Geometry: final body of the model. Coordinates: model frame, mm. A direction names the side the tool comes from. Round coordinates to 2 decimals unless told otherwise and drop trailing zeros. Loops run counter-clockwise (first coordinate to the right, second up) from the corner with the lowest first, then second, coordinate; pieces in that order, holes last. Notation, with made-up numbers: (19.25, 77) - (23.25, 77) arc R37 cw to (23.25, 116) - close; hole circle Ø4 at (54.25, -4). An arc over 180 degrees is marked (long way). Answer as CSV lines item,"result".
from build123d import *

# Parameters (mm, degrees)
SKETCH1_R           = 10.5
SKETCH1_R_2         = 1.5
BOSS_EXTRUDE1_DEPTH = 2.5
SKETCH2_R           = 4.5
SKETCH2_R_2         = 2.5
BOSS_EXTRUDE2_DEPTH = 3
CUT_EXTRUDE1_REACH  = 17.835
SKETCH3_R           = 1


with BuildPart() as part:
    # Sketch1 → Boss-Extrude1 (new body)
    with BuildSketch(Plane(origin=(0, 0, 0), x_dir=(1, 0, 0), z_dir=(0, 1, 0))):
        with Locations(Location((0, 0, 0), (0, 0, 270))):
            Circle(SKETCH1_R)
        with Locations(Location((0, 0, 0), (0, 0, 270))):
            Circle(SKETCH1_R_2, mode=Mode.SUBTRACT)
    extrude(amount=BOSS_EXTRUDE1_DEPTH)

    # Sketch2 → Boss-Extrude2 (add)
    with BuildSketch(Plane(origin=(0, 2.5, 0), x_dir=(1, 0, 0), z_dir=(0, 1, 0))):
        with Locations(Location((0, 0, 0), (0, 0, 270))):
            Circle(SKETCH2_R)
        with Locations(Location((0, 0, 0), (0, 0, 270))):
            Circle(SKETCH2_R_2, mode=Mode.SUBTRACT)
    extrude(amount=BOSS_EXTRUDE2_DEPTH)

    # Sketch3 → Cut-Extrude1 (cut, up to next)
    with BuildSketch(Plane.XZ, mode=Mode.PRIVATE) as cut_extrude1_sk1:
        with Locations(Location((-3.5, 7, 0), (0, 0, 270))):
            Circle(SKETCH3_R)
    cut_extrude1_tool1 = extrude(cut_extrude1_sk1.sketch, amount=-CUT_EXTRUDE1_REACH, mode=Mode.PRIVATE) & part.part
    # Sketch3 → Cut-Extrude1 (cut, up to next)
    with BuildSketch(Plane.XZ, mode=Mode.PRIVATE) as cut_extrude1_sk2:
        with Locations(Location((0, 7, 0), (0, 0, 270))):
            Circle(SKETCH3_R)
    cut_extrude1_tool2 = extrude(cut_extrude1_sk2.sketch, amount=-CUT_EXTRUDE1_REACH, mode=Mode.PRIVATE) & part.part
    # Sketch3 → Cut-Extrude1 (cut, up to next)
    with BuildSketch(Plane.XZ, mode=Mode.PRIVATE) as cut_extrude1_sk3:
        with Locations(Location((3.5, 7, 0), (0, 0, 270))):
            Circle(SKETCH3_R)
    cut_extrude1_tool3 = extrude(cut_extrude1_sk3.sketch, amount=-CUT_EXTRUDE1_REACH, mode=Mode.PRIVATE) & part.part
    # Sketch3 → Cut-Extrude1 (cut, up to next)
    with BuildSketch(Plane.XZ, mode=Mode.PRIVATE) as cut_extrude1_sk4:
        with Locations(Location((7, -3.5, 0), (0, 0, 270))):
            Circle(SKETCH3_R)
    cut_extrude1_tool4 = extrude(cut_extrude1_sk4.sketch, amount=-CUT_EXTRUDE1_REACH, mode=Mode.PRIVATE) & part.part
    # Sketch3 → Cut-Extrude1 (cut, up to next)
    with BuildSketch(Plane.XZ, mode=Mode.PRIVATE) as cut_extrude1_sk5:
        with Locations(Location((7, 0, 0), (0, 0, 270))):
            Circle(SKETCH3_R)
    cut_extrude1_tool5 = extrude(cut_extrude1_sk5.sketch, amount=-CUT_EXTRUDE1_REACH, mode=Mode.PRIVATE) & part.part
    # Sketch3 → Cut-Extrude1 (cut, up to next)
    with BuildSketch(Plane.XZ, mode=Mode.PRIVATE) as cut_extrude1_sk6:
        with Locations(Location((7, 3.5, 0), (0, 0, 270))):
            Circle(SKETCH3_R)
    cut_extrude1_tool6 = extrude(cut_extrude1_sk6.sketch, amount=-CUT_EXTRUDE1_REACH, mode=Mode.PRIVATE) & part.part
    # Sketch3 → Cut-Extrude1 (cut, up to next)
    with BuildSketch(Plane.XZ, mode=Mode.PRIVATE) as cut_extrude1_sk7:
        with Locations(Location((-3.5, -7, 0), (0, 0, 270))):
            Circle(SKETCH3_R)
    cut_extrude1_tool7 = extrude(cut_extrude1_sk7.sketch, amount=-CUT_EXTRUDE1_REACH, mode=Mode.PRIVATE) & part.part
    # Sketch3 → Cut-Extrude1 (cut, up to next)
    with BuildSketch(Plane.XZ, mode=Mode.PRIVATE) as cut_extrude1_sk8:
        with Locations(Location((0, -7, 0), (0, 0, 270))):
            Circle(SKETCH3_R)
    cut_extrude1_tool8 = extrude(cut_extrude1_sk8.sketch, amount=-CUT_EXTRUDE1_REACH, mode=Mode.PRIVATE) & part.part
    # Sketch3 → Cut-Extrude1 (cut, up to next)
    with BuildSketch(Plane.XZ, mode=Mode.PRIVATE) as cut_extrude1_sk9:
        with Locations(Location((3.5, -7, 0), (0, 0, 270))):
            Circle(SKETCH3_R)
    cut_extrude1_tool9 = extrude(cut_extrude1_sk9.sketch, amount=-CUT_EXTRUDE1_REACH, mode=Mode.PRIVATE) & part.part
    # Sketch3 → Cut-Extrude1 (cut, up to next)
    with BuildSketch(Plane.XZ, mode=Mode.PRIVATE) as cut_extrude1_sk10:
        with Locations(Location((-7, 3.5, 0), (0, 0, 270))):
            Circle(SKETCH3_R)
    cut_extrude1_tool10 = extrude(cut_extrude1_sk10.sketch, amount=-CUT_EXTRUDE1_REACH, mode=Mode.PRIVATE) & part.part
    # Sketch3 → Cut-Extrude1 (cut, up to next)
    with BuildSketch(Plane.XZ, mode=Mode.PRIVATE) as cut_extrude1_sk11:
        with Locations(Location((-7, 0, 0), (0, 0, 270))):
            Circle(SKETCH3_R)
    cut_extrude1_tool11 = extrude(cut_extrude1_sk11.sketch, amount=-CUT_EXTRUDE1_REACH, mode=Mode.PRIVATE) & part.part
    # Sketch3 → Cut-Extrude1 (cut, up to next)
    with BuildSketch(Plane.XZ, mode=Mode.PRIVATE) as cut_extrude1_sk12:
        with Locations(Location((-7, -3.5, 0), (0, 0, 270))):
            Circle(SKETCH3_R)
    cut_extrude1_tool12 = extrude(cut_extrude1_sk12.sketch, amount=-CUT_EXTRUDE1_REACH, mode=Mode.PRIVATE) & part.part
    add(cut_extrude1_tool1.solids().sort_by_distance((-3.5, 0, 7))[0], mode=Mode.SUBTRACT)
    add(cut_extrude1_tool2.solids().sort_by_distance((0, 0, 7))[0], mode=Mode.SUBTRACT)
    add(cut_extrude1_tool3.solids().sort_by_distance((3.5, 0, 7))[0], mode=Mode.SUBTRACT)
    add(cut_extrude1_tool4.solids().sort_by_distance((7, 0, -3.5))[0], mode=Mode.SUBTRACT)
    add(cut_extrude1_tool5.solids().sort_by_distance((7, 0, 0))[0], mode=Mode.SUBTRACT)
    add(cut_extrude1_tool6.solids().sort_by_distance((7, 0, 3.5))[0], mode=Mode.SUBTRACT)
    add(cut_extrude1_tool7.solids().sort_by_distance((-3.5, 0, -7))[0], mode=Mode.SUBTRACT)
    add(cut_extrude1_tool8.solids().sort_by_distance((0, 0, -7))[0], mode=Mode.SUBTRACT)
    add(cut_extrude1_tool9.solids().sort_by_distance((3.5, 0, -7))[0], mode=Mode.SUBTRACT)
    add(cut_extrude1_tool10.solids().sort_by_distance((-7, 0, 3.5))[0], mode=Mode.SUBTRACT)
    add(cut_extrude1_tool11.solids().sort_by_distance((-7, 0, 0))[0], mode=Mode.SUBTRACT)
    add(cut_extrude1_tool12.solids().sort_by_distance((-7, 0, -3.5))[0], mode=Mode.SUBTRACT)


solid = part.part
(1) Section B-B (y = 2.1). Give the number of separate pieces and of enclosed holes in the cut face, and give its area (3 significant figures).
Findings below:
separate pieces,"1"
enclosed holes,"13"
area,"302 mm2"
(2) Pin query (flat end, axial travel): P1, Ø2.5, axis at x = -3.5, z = -7, coming from the +Y side; P2, Ø1.5, axis at x = 1.5, y = 4, coming from the +Z side. Return the tip coordinate at first contact, or that it passes through.
Findings below:
P1,"y = 2.5"
P2,"z = 4.44"
(3) Section C-C (x = 0). Output: boundary loops of the cut face in (y, z), and give its area (3 significant figures).
Findings below:
outline,"(0, -10.5) - (2.5, -10.5) - (2.5, -8) - (0, -8) - close; (0, -6) - (2.5, -6) - (2.5, -4.5) - (5.5, -4.5) - (5.5, -2.5) - (2.5, -2.5) - (2.5, -1.5) - (0, -1.5) - close; (0, 1.5) - (2.5, 1.5) - (2.5, 2.5) - (5.5, 2.5) - (5.5, 4.5) - (2.5, 4.5) - (2.5, 6) - (0, 6) - close; (0, 8) - (2.5, 8) - (2.5, 10.5) - (0, 10.5) - close"
area,"47.0 mm2"
(4) Section A-A (z = 0). Output: boundary loops of the cut face in (x, y), and give its area (3 significant figures).
Findings below:
outline,"(-10.5, 0) - (-8, 0) - (-8, 2.5) - (-10.5, 2.5) - close; (-6, 0) - (-1.5, 0) - (-1.5, 2.5) - (-2.5, 2.5) - (-2.5, 5.5) - (-4.5, 5.5) - (-4.5, 2.5) - (-6, 2.5) - close; (1.5, 0) - (6, 0) - (6, 2.5) - (4.5, 2.5) - (4.5, 5.5) - (2.5, 5.5) - (2.5, 2.5) - (1.5, 2.5) - close; (8, 0) - (10.5, 0) - (10.5, 2.5) - (8, 2.5) - close"
area,"47.0 mm2"
(5) Access query for faces 1 (the face through (-2, 2.5, 0)), 2 (the face through (-2, 5.5, 2)). Directions: +Z, -Z, +X, -X, +Y, -Y. A direction counts if a zero-diameter tool reaches every point of the face in a straight line with its end or side. Return the directions, or none.
Findings below:
face 1,"+Y"
face 2,"+Z, -Z, +X, -X, +Y"
(6) Draft query along X for faces 3 (the face through (3.2, 1.2, 10)), 4 (the face through (0, 2.5, 5)), 5 (the face through (0.45, 1.23, 1.43)). Return one class per face: pulls with the +X half, pulls with the -X half, needs draft (parallel to the pull), parting line crosses it, or undercut.
Findings below:
face 3,"parting line crosses it"
face 4,"needs draft"
face 5,"undercut"
(7) Material intervals for line 1 along X through (y, z) = (1.55, 0); line 2 along X through (y, z) = (0.75, 7); line 3 along X through (y, z) = (1.45, 3.5), sorted ascending.
Findings below:
line 1,"-10.5 to -8, -6 to -1.5, 1.5 to 6, 8 to 10.5"
line 2,"-7.83 to -4.5, -2.5 to -1, 1 to 2.5, 4.5 to 7.83"
line 3,"-9.9 to -8, -6 to 6, 8 to 9.9"
(8) Section D-D (x = -3.5). Output: boundary loops of the cut face in (y, z), and give its area (3 significant figures).
Findings below:
outline,"(0, -9.9) - (2.5, -9.9) - (2.5, -8) - (0, -8) - close; (0, -6) - (2.5, -6) - (2.5, -2.83) - (5.5, -2.83) - (5.5, 2.83) - (2.5, 2.83) - (2.5, 6) - (0, 6) - close; (0, 8) - (2.5, 8) - (2.5, 9.9) - (0, 9.9) - close"
area,"56.5 mm2"
